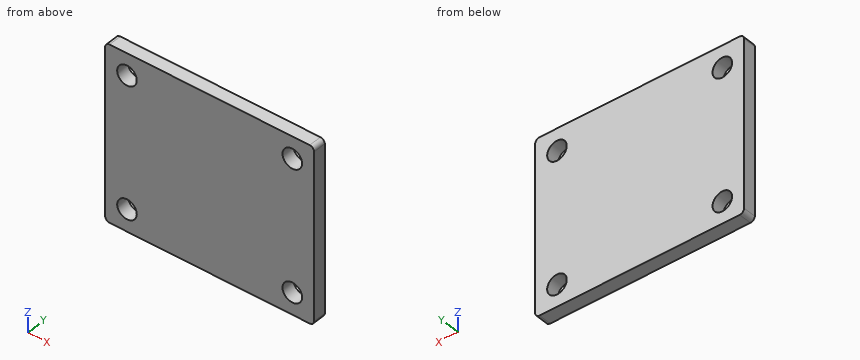
from build123d import *

# Parameters (mm, degrees)
F0_R     = 7.14375
F1_DEPTH = 4.7625


with BuildPart() as f1:
    # F0 (on Front) → F1 (new body, symmetric)
    with BuildSketch(Plane.XZ):
        with BuildLine():
            Line((-73.025, -63.5), (73.025, -63.5))
            ThreePointArc((73.025, -63.5), (75.270064, -62.570064), (76.2, -60.325))
            Line((76.2, -60.325), (76.2, 60.325))
            ThreePointArc((76.2, 60.325), (75.270064, 62.570064), (73.025, 63.5))
            Line((73.025, 63.5), (-73.025, 63.5))
            ThreePointArc((-73.025, 63.5), (-75.270064, 62.570064), (-76.2, 60.325))
            Line((-76.2, 60.325), (-76.2, -60.325))
            ThreePointArc((-76.2, -60.325), (-75.270064, -62.570064), (-73.025, -63.5))
        make_face()
        with Locations((-60.325, -47.625)):
            Circle(F0_R, mode=Mode.SUBTRACT)
        with Locations((60.325, -47.625)):
            Circle(F0_R, mode=Mode.SUBTRACT)
        with Locations((-60.325, 47.625)):
            Circle(F0_R, mode=Mode.SUBTRACT)
        with Locations((60.325, 47.625)):
            Circle(F0_R, mode=Mode.SUBTRACT)
    extrude(amount=F1_DEPTH, both=True)


solid = f1.part
The listing builds one solid part. Answer for the finished solid, in the listing's coordinates (mm). Round coordinates to 2 decimals unless told otherwise and drop trailing zeros. Write each loop counter-clockwise with the first axis right and the second up, starting at its lowest first coordinate (ties: lowest second). Pieces come first, ordered by that corner, then holes. Notation, with made-up numbers: (76.5, -32) - (98.5, -32) arc R21 ccw to (98.5, -24) - close; hole circle Ø1 at (77, 44). An arc over 180 degrees is marked (long way). Use one line per item in the form item = value. Start each with the question number.
Item 1: A cutting plane is placed at B-B (y = 1). Give the number of separate pieces and of enclosed holes in the cut face, plus the area to 3 significant figures.
Item 2: Flat-ended cylindrical pins translate along their axes: pin 1 Ø18.5 at (x, z) = (-60.325, 47.625) entering from -Y; pin 2 Ø13 at (x, z) = (60.325, 47.625) entering from +Y. Find the tip coordinate at first contact, or state that the pin passes through.
Item 3: A cutting plane is placed at A-A (x = -64). Write down the section's boundary in (y, z), plus the area to 3 significant figures.
Item 4: Find the intervals of material crossed by line 1 (X direction, y = -2.5, z = -51.5); line 2 (X direction, y = -1.25, z = 46), in increasing order. Write a range as [from, to].
The answers:
q1.separate_pieces = 1
q1.enclosed_holes = 4
q1.area = 18,700 mm^2
q2.pin_1 = -4.76
q2.pin_2 = through
q3.outline = (-4.76, -63.5) - (4.76, -63.5) - (4.76, -53.75) - (-4.76, -53.75) - close; (-4.76, -41.5) - (4.76, -41.5) - (4.76, 41.5) - (-4.76, 41.5) - close; (-4.76, 53.75) - (4.76, 53.75) - (4.76, 63.5) - (-4.76, 63.5) - close
q3.area = 976 mm^2
q4.line_1 = [-76.2, -66.33], [-54.32, 54.32], [66.33, 76.2]
q4.line_2 = [-76.2, -67.28], [-53.37, 53.37], [67.28, 76.2]
